```python
from build123d import *

# Parameters (mm, degrees)
F0_R      = 24.4
F0_R_2    = 23.15
F1_DEPTH  = 22
F3_DEPTH  = 2.5
F4_W      = 9
F4_H      = 7
F5_DEPTH  = 25
F6_W      = 9
F6_H      = 7
F7_DEPTH  = 25
F8_W      = 9
F8_H      = 24.4
F9_DEPTH  = 25
F10_W     = 9
F10_H     = 24.4
F11_DEPTH = 25
F13_R     = 24.4
F12_R     = 24.4
F12_R_2   = 23.15
F14_DEPTH = 2.5
F15_R     = 18.25
F15_R_2   = 17.25
F16_DEPTH = 150
F17_R     = 17.5
F18_DEPTH = 25


with BuildPart() as f1:
    # F0 (on Front) → F1 (new body)
    with BuildSketch(Plane.XZ):
        Circle(F0_R)
        Circle(F0_R_2, mode=Mode.SUBTRACT)
    extrude(amount=-F1_DEPTH)

    # F2 (on Front) → F3 (join)
    with BuildSketch(Plane.XZ):
        with BuildLine():
            Line((15, 16.77051), (15, 34.914181))
            ThreePointArc((15, 34.914181), (0, 38), (-15, 34.914181))
            Line((-15, 34.914181), (-15, 16.77051))
            ThreePointArc((-15, 16.77051), (0, 22.5), (15, 16.77051))
        make_face()
    extrude(amount=F3_DEPTH)

    # F4 (on Right) → F5 (cut)
    with BuildSketch(Plane.YZ):
        with Locations((4.5, 13.5)):
            Rectangle(F4_W, F4_H)
    extrude(amount=-F5_DEPTH, mode=Mode.SUBTRACT)

    # F6 (on Right) → F7 (cut)
    with BuildSketch(Plane.YZ):
        with Locations((4.5, 13.5)):
            Rectangle(F6_W, F6_H)
    extrude(amount=F7_DEPTH, mode=Mode.SUBTRACT)

    # F8 (on Right) → F9 (cut)
    with BuildSketch(Plane.YZ):
        with Locations((4.5, -12.2)):
            Rectangle(F8_W, F8_H)
    extrude(amount=-F9_DEPTH, mode=Mode.SUBTRACT)

    # F10 (on Right) → F11 (cut)
    with BuildSketch(Plane.YZ):
        with Locations((4.5, -12.2)):
            Rectangle(F10_W, F10_H)
    extrude(amount=F11_DEPTH, mode=Mode.SUBTRACT)

    # F13 (on face) + F12 (on face) → F14 (join)
    with BuildSketch(Plane(origin=(0, 22, 0), x_dir=(-1, 0, 0), z_dir=(0, 1, 0))):
        Circle(F13_R)
    with BuildSketch(Plane(origin=(0, 22, 0), x_dir=(-1, 0, 0), z_dir=(0, 1, 0))):
        Circle(F12_R)
        Circle(F12_R_2, mode=Mode.SUBTRACT)
    extrude(amount=F14_DEPTH)

    # F15 (on face) → F16 (join)
    with BuildSketch(Plane(origin=(0, 24.5, 0), x_dir=(-1, 0, 0), z_dir=(0, 1, 0))):
        Circle(F15_R)
        Circle(F15_R_2, mode=Mode.SUBTRACT)
    extrude(amount=F16_DEPTH)

    # F17 (on face) → F18 (cut)
    with BuildSketch(Plane.XZ.offset(-22)):
        Circle(F17_R)
    extrude(amount=-F18_DEPTH, mode=Mode.SUBTRACT)


solid = f1.part
```
Design review of the part built by this model. Coordinates are the model's own, in mm. A direction names the side the tool comes from. Coordinates: 2 decimals unless noted, no trailing zeros. Write each loop counter-clockwise with the first axis right and the second up, starting at its lowest first coordinate (ties: lowest second). Pieces come first, ordered by that corner, then holes. Notation, with made-up numbers: M -15.5,-32 L 4.5,-32 A15 cw 4.5,-6 Z; hole C 8,27 d10. An arc over 180 degrees is marked long. Answer as a JSON object with one key per item and string values.
Item 1: Add section C-C, the plane x = 9. Give the boundary of the cut face in (y, z).
Outcome:
{"outline": "M -2.5,20.62 L 0,20.62 L 0,21.33 L 22,21.33 L 22,15.01 L 47,15.01 L 47,14.72 L 174.5,14.72 L 174.5,15.88 L 24.5,15.88 L 24.5,22.68 L 0,22.68 L 0,36.92 L -2.5,36.92 Z; M 9,-22.68 L 24.5,-22.68 L 24.5,-15.88 L 174.5,-15.88 L 174.5,-14.72 L 47,-14.72 L 47,-15.01 L 22,-15.01 L 22,-21.33 L 9,-21.33 Z"}
Item 2: Add section D-D, the plane y = 31.5. Give the boundary of the cut face in (x, z), and give its area (3 significant figures).
Outcome:
{"outline": "C 0,0 d36.5; hole C 0,0 d35", "area": "84.2 mm²"}
Item 3: Add section B-B, the plane y = 53. Give the boundary of the cut face in (x, z).
Outcome:
{"outline": "C 0,0 d36.5; hole C 0,0 d34.5"}
Item 4: Machinability: for faces 5 (the cylindrical face through (-13.887, 34.325, -10.648)), 6 (the flat face through (23, 0, 5)), 7 (the flat face through (-19, 9, 14)), 8 (the cylindrical face through (-3.014, 13.29, 22.953)), 9 (the cylindrical face through (0, -1, 38)), which of the approach directions +Z, -Z, +X, -X, +Y, -Y give a long, thin tool a straight path to every point of the face, cutting with its end or side? Answer none if there is none.
Outcome:
{"face 5": "-Y", "face 6": "+Z, -Z, +X, -X, -Y", "face 7": "+X, -X, -Y", "face 8": "none", "face 9": "+Z, +Y, -Y"}
Item 5: Add section A-A, the plane x = 0. Give the boundary of the cut face in (y, z), and give its area (3 significant figures).
Outcome:
{"outline": "M -2.5,22.5 L 0,22.5 L 0,23.15 L 22,23.15 L 22,17.5 L 47,17.5 L 47,17.25 L 174.5,17.25 L 174.5,18.25 L 24.5,18.25 L 24.5,24.4 L 0,24.4 L 0,38 L -2.5,38 Z; M 9,-24.4 L 24.5,-24.4 L 24.5,-18.25 L 174.5,-18.25 L 174.5,-17.25 L 47,-17.25 L 47,-17.5 L 22,-17.5 L 22,-23.15 L 9,-23.15 Z", "area": "406 mm²"}
Item 6: Wall thickness on probe 1 along Z at (x, y) = (0, 30); probe 2 along Z at (x, y) = (0, 133); probe 3 along X at (y, z) = (114, -7): over which ranges is each line inside the solid? List them lowest first.
Outcome:
{"probe 1": "-18.25 to -17.5, 17.5 to 18.25", "probe 2": "-18.25 to -17.25, 17.25 to 18.25", "probe 3": "-16.85 to -15.77, 15.77 to 16.85"}
Item 7: Draft analysis for pull direction X (two halves, no side actions). For faces 1 (the cylindrical face through (-0.2, -1.2, 22.5)), 2 (the flat face through (-0.1, 0, 22.8)), 3 (the flat face through (-4, 9, -23)), 4 (the cylindrical face through (3.956, 98.45, -17.816)), state which applies: pulls with the +X half, pulls with the -X half, needs draft (parallel to the pull), parting line crosses it, or undercut.
Outcome:
{"face 1": "undercut", "face 2": "undercut", "face 3": "needs draft", "face 4": "parting line crosses it"}
Item 8: Insertion check: pin 1 Ø12 at (y, z) = (155.5, 6.5) entering from +X; pin 2 Ø1.1 at (x, z) = (22, 3) entering from -Y; pin 3 Ø2 at (y, z) = (-1.5, 27.5) entering from -X. Each pin has a flat end and moves straight along its axis. Give the tip position at first contact, or say it passes through.
Outcome:
{"pin 1": "x = 18.24", "pin 2": "y = 22", "pin 3": "x = -15"}
